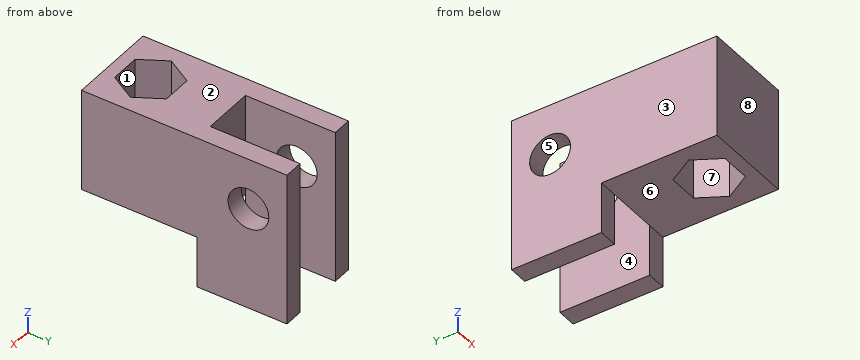
```python
from build123d import *

# Parameters (mm, degrees)
BOSS_EXTRUDE1_DEPTH     = 25.4
CUT_EXTRUDE1_DEPTH      = 26.4
F_3_8_CLEARANCE_HOLE1_D = 10.0838
SKETCH7_W               = 4.7625
SKETCH7_H               = 22.225
BOSS_EXTRUDE2_DEPTH     = 12.7


with BuildPart() as part:
    # Sketch1 → Boss-Extrude1 (new body)
    with BuildSketch(Plane.XY):
        Polygon((-11.1125, 0), (11.1125, 0), (11.1125, 50.8), (6.35, 50.8), (6.35, 28.575), (-6.35, 28.575), (-6.35, 50.8), (-11.1125, 50.8), align=None)
    extrude(amount=BOSS_EXTRUDE1_DEPTH)

    # Sketch2 → Cut-Extrude1 (cut, through all)
    with BuildSketch(Plane.XY.offset(25.4)):
        Polygon((3.702835951, 15.9385), (-3.702835951, 15.9385), (-7.405671903, 9.525), (-3.702835951, 3.1115), (3.702835951, 3.1115), (7.405671903, 9.525), align=None)
    extrude(amount=-CUT_EXTRUDE1_DEPTH, mode=Mode.SUBTRACT)

    # 3/8 Clearance Hole1 (through all)
    with Locations(Plane.ZY.offset(11.1125)):
        with Locations((12.7, 41.275)):
            Hole(F_3_8_CLEARANCE_HOLE1_D / 2)

    # Sketch7 → Boss-Extrude2 (add)
    with BuildSketch(Plane(origin=(0, 0, 0), x_dir=(-1, 0, 0), z_dir=(0, 0, -1))):
        with Locations((-8.73125, 39.6875)):
            Rectangle(SKETCH7_W, SKETCH7_H)
        with Locations((8.73125, 39.6875)):
            Rectangle(SKETCH7_W, SKETCH7_H)
    extrude(amount=BOSS_EXTRUDE2_DEPTH)


solid = part.part
```
Build history of the part. All positions in model axes, mm. Face numbers are marked on the shaded views. A direction names the side the tool comes from. Give positions to 0.01 mm unless a question says otherwise; leave off trailing zeros. Loops run counter-clockwise (first coordinate to the right, second up) from the corner with the lowest first, then second, coordinate; pieces in that order, holes last.
Item 1: Which spindle directions (+Z, -Z, +X, -X, +Y, -Y) get a long thin tool onto all of the face, cutting with end or side? Do the marked faces 4, 5, 6, 7 and 8. Say none if no direction does.
Answers follow:
face 4: +Z, -Z, +Y
face 5: +X, -X
face 6: -Z, +X, -X, -Y
face 7: +Z, -Z
face 8: +Z, -Z, +X, -X, -Y
Item 2: Slice it at C-C, the plane x = -5.75. List the corners of the cut face in (y, z) (3 decimals).
Answers follow:
outline: (0, 0) - (6.657, 0) - (6.657, 25.4) - (0, 25.4) - close; (12.393, 0) - (28.575, 0) - (28.575, 25.4) - (12.393, 25.4) - close
Item 3: Slice it at A-A, the plane z = 12.7. Give the number of separate pieces and of enclosed holes in the cut face, and give its area (3 significant figures).
Answers follow:
separate pieces: 3
enclosed holes: 1
area: 608 mm2
Item 4: Drill centre lines: line 1 (X direction, y = 41.5, z = 18.5); line 2 (Y direction, x = 7.45, z = 12.7). Where is each one in solid material? Low to high.
Answers follow:
line 1: x = -11.11 to -6.35, 6.35 to 11.11
line 2: y = 0 to 36.23, 46.32 to 50.8
Item 5: Pull direction X, two halves, no side cores. Call the marked faces 1, 2 and 3: released by +X, released by -X, zero draft, split by the parting line, or undercut.
Answers follow:
face 1: undercut
face 2: zero draft
face 3: released by -X
Item 6: Flat gauge pins, fed straight in: pin 1 (2.5 mm diameter, centred on x = -9.5, z = -8.5, fed in from -Y) (3 decimals); pin 2 (1 mm diameter, centred on x = 2, y = 30, fed in from -Z); pin 3 (10 mm diameter, centred on x = 0, z = 10.5, fed in from +Y) (3 decimals); pin 4 (1 mm diameter, centred on x = 7, y = 24, fed in from -Z). Where does each tip first touch, or does it go through?
Answers follow:
pin 1: stops at y = 28.575
pin 2: passes through
pin 3: stops at y = 28.575
pin 4: stops at z = 0
